Autodesk Inventor part; units mm, degrees
ref_plane "作業平面1" through (18.75, 8.39, -7.25) normal (1, 0, 0) x (0, 1, 0)
ref_plane "YZ Plane" through (0, 0, 0) normal (1, 0, 0) x (0, 1, 0)
ref_plane "XZ Plane" through (0, 0, 0) normal (0, 1, 0) x (-1, 0, 0)
sketch "スケッチ1" plane through (0, 0, 0) normal (0, 1, 0) x (-1, 0, 0)
  line L0 (21.5, -48.5) -> (-21.5, -48.5)
  line L1 (-21.5, -48.5) -> (-21.5, 48.5)
  line L2 (-21.5, 48.5) -> (21.5, 48.5)
  line L3 (21.5, 48.5) -> (21.5, -48.5)
  line L4 (21.5, -48.5) -> (-21.5, 48.5) construction
  line L5 (-21.5, -48.5) -> (21.5, 48.5) construction
  point P0 (0, 0)
  dimension "d0" = 43
  dimension "d1" = 97
extrude "押し出し1" add sketch "スケッチ1" along normal blind 14
shell "シェル1" thickness 1.5 removed faces 1 at (-7.1667, 14, -16.1667)
fillet "フィレット1" radius 5 4 edges at (-21.5, 0, 0) (21.5, 0, 0) (-20, 1.5, 0) (20, 1.5, 0)
sketch "スケッチ2" plane through (21.5, 14, -48.5) normal (0, 0, -1) x (-1, 0, 0)
  arc A0 (1.5, -7.5) -> (6.5, -12.5) centre (6.5, -7.5) ccw
  line L0 (1.5, -7.5) -> (1.5, 0)
  line L1 (41.5, 0) -> (1.5, 0)
  line L2 (41.5, -7.5) -> (41.5, 0)
  arc A1 (36.5, -12.5) -> (41.5, -7.5) centre (36.5, -7.5) ccw
  line L3 (6.5, -12.5) -> (36.5, -12.5)
  line L4 (1.5, -4.5) -> (41.5, -4.5)
  line L5 (9, -4.5) -> (34, -4.5)
  line L6 (34, -4.5) -> (34, -12.5)
  line L7 (34, -12.5) -> (9, -12.5)
  line L8 (9, -12.5) -> (9, -4.5)
  point P0 (21.5, -14)
  point P1 (21.5, -4.5)
  point P2 (9, -12.5)
  dimension "d8" = 8
  dimension "d9" = 25
extrude "押し出し2" cut sketch "スケッチ2" against normal up to surface (1.5 mm away) contours L8 L4 L6 L3
sketch "スケッチ3" plane through (0, 0, 0) normal (0, -1, 0) x (1, 0, 0)
  circle A0 centre (0, 51.5) radius 3
  circle A1 centre (24.5, -45.5) radius 3
  circle A2 centre (-24.5, -45.5) radius 3
  line L0 (-21.5, 48.5) -> (-21.5, -48.5)
  line L1 (16.5, -48.5) -> (-16.5, -48.5)
  line L2 (21.5, -48.5) -> (21.5, 48.5)
  line L3 (-16.5, 48.5) -> (16.5, 48.5)
  line L4 (-24.5, -48.5) -> (24.5, -48.5)
  arc A3 (21.5, 48.5) -> (-21.5, 48.5) centre (0, 12.9792) ccw
  line L5 (-21.5, 48.5) -> (-16.5, 48.5)
  line L6 (16.5, 48.5) -> (21.5, 48.5)
  circle A4 centre (0, 51.5) radius 1.6
  circle A5 centre (24.5, -45.5) radius 1.6
  circle A6 centre (-24.5, -45.5) radius 1.6
  point P0 (0, 0)
  point P1 (-21.5, -45.5)
  point P2 (21.5, -45.5)
  dimension "d11" = 6
  dimension "d12" = 6
  dimension "d10" = 6
  dimension "d13" = 3.2
  dimension "d14" = 3.2
  dimension "d15" = 3.2
extrude "押し出し3" add sketch "スケッチ3" against normal up to surface (14 mm away) contours A0 | A0 A3 L6 L3 | A0 L3 L5 A3 | A1 | A1 L4 L2 | A2 | L0 L4 A2
extrude "押し出し4" cut sketch "スケッチ3" against normal blind 11 contours A0 | A0 A3 L6 L3 | A0 L3 L5 A3 | A1 | A1 L4 L2 | A2 | L0 L4 A2 | A4 | A6
fillet "フィレット2" radius 5 2 edges at (-21.5, 12.5, -45.5) (21.5, 12.5, -45.5)
sketch "スケッチ4" plane through (21.5, 5, 48.5) normal (1, 0, 0) x (0, 0, -1)
  line L0 (20, 9) -> (45, 9)
  line L1 (45, 9) -> (45, -1)
  line L2 (45, -1) -> (20, -1)
  line L3 (20, -1) -> (20, 9)
  line L4 (0, 9) -> (86.254, 9)
  line L5 (0, 0) -> (0, 6)
  point P0 (48.5, -5)
  dimension "d21" = 25
  dimension "d22" = 10
  dimension "d23" = 20
extrude "押し出し5" add sketch "スケッチ4" along normal blind 5
sketch "スケッチ5" plane through (26.5, 5, 48.5) normal (1, 0, 0) x (0, 0, -1)
  circle A0 centre (26, 4) radius 1.3
  circle A1 centre (39, 4) radius 1.3
  line L0 (20, 9) -> (20, -1)
  line L1 (45, -1) -> (45, 9)
  point P0 (48.5, -5)
  point P1 (20, 4)
  dimension "d26" = 2.6
  dimension "d27" = 2.6
  dimension "d28" = 6
  dimension "d29" = 6
ref_plane "作業平面1" through (18.75, 8.39, -7.25) normal (1, 0, 0) x (0, 1, 0)
extrude "押し出し6" cut sketch "スケッチ5" against normal up to surface (7.75 mm away)
sketch "スケッチ6" plane through (21.5, 4, 28.5) normal (0, 0, 1) x (1, 0, 0)
  arc A0 (-5, -4) -> (0, 1) centre (-5, 1) ccw
  line L0 (0, 0) -> (5, 0)
  line L1 (0, 1) -> (0, 0)
  line L2 (0, 0) -> (-0.101, 0)
  point P0 (-21.5, -4)
extrude "押し出し7" add sketch "スケッチ6" against normal up to surface (25 mm away)
properties part number "handle_monitor_case_under"
Source: CAD feature listing. Evaluate the final solid. Frame: model axes, mm. A direction names the side the tool comes from. Round coordinates to 2 decimals unless told otherwise and drop trailing zeros. Loops run counter-clockwise (first coordinate to the right, second up) from the corner with the lowest first, then second, coordinate; pieces in that order, holes last.
(1) Section query C-C (z = 36). Output: boundary loops of the cut face in (x, y), and give its area (3 significant figures).
From the geometry:
outline: (-21.5, 5) arc R5 ccw to (-16.5, 0) - (16.5, 0) arc R5 ccw to (21.5, 5) - (21.5, 14) - (20, 14) - (20, 6.5) arc R5 cw to (15, 1.5) - (-15, 1.5) arc R5 cw to (-20, 6.5) - (-20, 14) - (-21.5, 14) - close
area: 102 mm2
(2) Section query B-B (z = 51.5). Output: boundary loops of the cut face in (x, y).
From the geometry:
outline: (-15.5, 11) - (-1.6, 11) - (-1.6, 14) - (-15.5, 14) - close; (1.6, 11) - (15.5, 11) - (15.5, 14) - (1.6, 14) - close
(3) Pull-direction query (X, two-part tool) for faces 1 (the cylindrical face through (-20, 1.43, -0.68)), 2 (the flat face through (21.5, 9, -23)), 3 (the flat face through (24, 4, 16)), 4 (the flat face through (0, 10, -47)); classes: +X half, -X half, draft (parallel to the pull), parting line (faces both ways), or undercut.
From the geometry:
face 1: -X half
face 2: +X half
face 3: draft
face 4: undercut
(4) Section query D-D (z = 13). Output: boundary loops of the cut face in (x, y), and give its area (3 significant figures).
From the geometry:
outline: (-21.5, 5) arc R5 ccw to (-16.5, 0) - (16.5, 0) arc R5 ccw to (21.4, 4) - (26.5, 4) - (26.5, 14) - (20, 14) - (20, 6.5) arc R5 cw to (15, 1.5) - (-15, 1.5) arc R5 cw to (-20, 6.5) - (-20, 14) - (-21.5, 14) - close
area: 152 mm2
(5) Access query for faces 5 (the cylindrical face through (-23.76, 12.48, -46.92)), 6 (the flat face through (-23, 11, -44)), 7 (the flat face through (24, 9, 28.5)), 8 (the flat face through (-20, 10, 1)), 9 (the flat face through (0, 5, 48.5)). Directions: +Z, -Z, +X, -X, +Y, -Y. A direction counts if a zero-diameter tool reaches every point of the face in a straight line with its end or side. Return the directions, or none.
From the geometry:
face 5: +Y, -Y
face 6: +Z, -Z, -X, -Y
face 7: +Z, +X, +Y, -Y
face 8: +Y
face 9: +Z, +X, -X, -Y
(6) Section query A-A (z = -45.5). Output: boundary loops of the cut face in (x, y).
From the geometry:
outline: (-27.5, 11) - (-26.1, 11) - (-26.1, 14) - (-27.5, 14) - close; (-22.9, 11) - (-21.5, 11) - (-21.5, 5) arc R5 ccw to (-16.5, 0) - (16.5, 0) arc R5 ccw to (21.5, 5) - (21.5, 11) - (22.9, 11) - (22.9, 14) - (20, 14) - (20, 6.5) arc R5 cw to (15, 1.5) - (-15, 1.5) arc R5 cw to (-20, 6.5) - (-20, 14) - (-22.9, 14) - close; (26.1, 11) - (27.5, 11) - (27.5, 14) - (26.1, 14) - close
(7) Contact query for flat-ended pins moving along their axis: pin 1 Ø6.5 at (x, z) = (-23.5, -44.5) entering from -Y; pin 2 Ø1.5 at (x, y) = (22.5, 9.5) entering from -Z; pin 3 Ø8 at (y, z) = (10.5, -7) entering from -X. Output: stop coordinate, or through.
From the geometry:
pin 1: stops at y = 1.69
pin 2: stops at z = 3.5
pin 3: stops at x = -21.5
(8) Material intervals for probe 1 along Z at (x, y) = (0, 13.3); probe 2 along Z at (x, y) = (18.5, 3); probe 3 along X at (y, z) = (11.5, -28), sorted ascending.
From the geometry:
probe 1: z = -48.5 to -47, 47 to 49.9, 53.1 to 54.5
probe 2: z = -48.5 to -47, 47 to 48.5
probe 3: x = -21.5 to -20, 20 to 21.5
